Build history of the part. All positions in model axes, mm. A direction names the side the tool comes from. Give positions to 0.01 mm unless a question says otherwise; leave off trailing zeros. Write each loop counter-clockwise with the first axis right and the second up, starting at its lowest first coordinate (ties: lowest second). Pieces come first, ordered by that corner, then holes. Notation, with made-up numbers: (-24.75, 74.25) -> (23.25, 74.25) arc R20 ccw to (23.25, 100.25) -> close; hole circle Ø1 at (57, 8). An arc over 180 degrees is marked (long way). One line per question, with ' | ' between items. Start each with the question number.
(1) Band-saw the part on C-C, the plane x = 3.75. Give the cut face in (y, z), and give its area (3 significant figures).
(2) Drill centre lines: probe 1 along Y at (x, z) = (3.6, -33); probe 2 along Y at (x, z) = (1, -14); probe 3 along Y at (x, z) = (1.25, -34). Where is each one in solid material? Low to high. Write a range as from..to.
(3) Pin check, flat tips, straight feed: P1, Ø8, axis at y = 6, z = -24.5, coming from the -X side; P2, Ø0.8, axis at x = -1, z = -28.5, coming from the +Y side (3 decimals); P3, Ø12, axis at y = 19.5, z = -19.5, coming from the -X side; P4, Ø4, axis at x = 1.5, z = -7, coming from the +Y side. Stop position of each tip, or through.
(4) Band-saw the part on B-B, the plane y = 38.75. Give the cut face in (x, z), and give its area (3 significant figures).
(5) Band-saw the part on A-A, the plane z = -33. Give the cut face in (x, y) (3 decimals), and give its area (3 significant figures).
(6) Band-saw the part on D-D, the plane z = -5. Give the cut face in (x, y) (3 decimals).
(7) Tool access for faces 1 (the flat face through (-1, 6.825, -7)), 2 (the flat face through (-1, 13.175, -7)), 3 (the flat face through (2, 10, 0)): list every direction of +Z, -Z, +X, -X, +Y, -Y with a clear straight run to the whole face (end or side of a thin tool).
from build123d import *

# Parameters (mm, degrees)
SKETCH1_R           = 1.5
BOSS_EXTRUDE1_DEPTH = 5
SKETCH3_W           = 40
SKETCH3_H           = 6.35
BOSS_EXTRUDE2_DEPTH = 2
FILLET1_R           = 0.5
FILLET2_R           = 3
SKETCH4_R           = 3.2004
CUT_EXTRUDE1_DEPTH  = 8
FILLET3_R           = 10


with BuildPart() as part:
    # Sketch1 → Boss-Extrude1 (new body)
    with BuildSketch(Plane(origin=(0, 0, 0), x_dir=(0, 0, -1), z_dir=(1, 0, 0))):
        Polygon((0, 0), (0, 20), (25, 20), (25, 44), (40, 44), (40, 0), align=None)
        with Locations((33, 38.75)):
            Circle(SKETCH1_R, mode=Mode.SUBTRACT)
        with Locations((33, 29.25)):
            Circle(SKETCH1_R, mode=Mode.SUBTRACT)
    extrude(amount=BOSS_EXTRUDE1_DEPTH)

    # Sketch3 → Boss-Extrude2 (add)
    with BuildSketch(Plane.ZY):
        with Locations((-20, 10)):
            Rectangle(SKETCH3_W, SKETCH3_H)
    extrude(amount=BOSS_EXTRUDE2_DEPTH)

    # Fillet1
    fillet1_edges = [part.edges().sort_by_distance(p)[0] for p in [
        (-2, 6.825, -20),
        (-2, 13.175, -20),
    ]]
    fillet(fillet1_edges, radius=FILLET1_R)

    # Fillet2
    fillet2_edges = [part.edges().sort_by_distance(p)[0] for p in [
        (2.5, 0, 0),
        (2.5, 20, 0),
        (2.5, 44, -25),
        (2.5, 0, -40),
    ]]
    fillet(fillet2_edges, radius=FILLET2_R)

    # Sketch4 → Cut-Extrude1 (cut, through all)
    with BuildSketch(Plane(origin=(5, 0, 0), x_dir=(0, 0, -1), z_dir=(1, 0, 0))):
        with Locations((14, 10)):
            Circle(SKETCH4_R)
    extrude(amount=-CUT_EXTRUDE1_DEPTH, mode=Mode.SUBTRACT)

    # Fillet3
    fillet3_edges = [part.edges().sort_by_distance(p)[0] for p in [
        (2.5, 20, -25),
    ]]
    fillet(fillet3_edges, radius=FILLET3_R)


solid = part.part
Results:
1) outline: (0, -37) arc R3 ccw to (3, -40) -> (44, -40) -> (44, -28) arc R3 ccw to (41, -25) -> (30, -25) arc R10 cw to (20, -15) -> (20, -3) arc R3 ccw to (17, 0) -> (3, 0) arc R3 ccw to (0, -3) -> close; hole circle Ø6.4 at (10, -14); hole circle Ø3 at (29.25, -33); hole circle Ø3 at (38.75, -33) | area: 1,130 mm²
2) probe 1: y = 0..27.75, 30.75..37.25, 40.25..44 | probe 2: y = 0..6.8, 13.2..20 | probe 3: y = 0..28.13, 30.37..37.63, 39.87..44
3) P1: stops at x = -2 | P2: stops at y = 13.175 | P3: stops at x = 0 | P4: stops at y = 20
4) outline: (0, -40) -> (5, -40) -> (5, -34.5) -> (0, -34.5) -> close; (0, -31.5) -> (5, -31.5) -> (5, -25) -> (0, -25) -> close | area: 60.0 mm²
5) outline: (-2, 7.325) arc R0.5 ccw to (-1.5, 6.825) -> (0, 6.825) -> (0, 0) -> (5, 0) -> (5, 27.75) -> (0, 27.75) -> (0, 13.175) -> (-1.5, 13.175) arc R0.5 ccw to (-2, 12.675) -> close; (0, 30.75) -> (5, 30.75) -> (5, 37.25) -> (0, 37.25) -> close; (0, 40.25) -> (5, 40.25) -> (5, 44) -> (0, 44) -> close | area: 203 mm²
6) outline: (-2, 7.325) arc R0.5 ccw to (-1.5, 6.825) -> (0, 6.825) -> (0, 0) -> (5, 0) -> (5, 20) -> (0, 20) -> (0, 13.175) -> (-1.5, 13.175) arc R0.5 ccw to (-2, 12.675) -> close
7) face 1: +Z, -Z, -X, -Y | face 2: +Z, -Z, -X, +Y | face 3: +Z, +X, -X, +Y, -Y
